Read the model definition and answer for the solid it produces. Units are mm, in the model's axes. A direction names the side the tool comes from. Give positions to 0.01 mm unless a question says otherwise; leave off trailing zeros. Order: outer loops, then holes, each group sorted by start corner. A loop starts at its lowest first (then second) coordinate and runs counter-clockwise, first axis right, second up. Notation, with made-up numbers: (2, -34) -> (47, -34) arc R15 ccw to (47, -26) -> close; hole circle Ø9 at (69.5, 20). An arc over 180 degrees is marked (long way). Answer as CSV lines item,"result". Start each with the question number.
1) Straight lines are drawn through the part: L1, parallel to Y at x = -25, z = 1.9; L2, parallel to X at y = -17, z = 1.35; L3, parallel to X at y = -18, z = 2.35. For each, find the intervals that lie inside material, in ascending order. Write a range as from..to.
2) Find section C-C (y = -26). Determine the outline of the cut face in (x, z).
3) Find section B-B (z = 2.45). State how many separate pieces and enclosed holes the cut face has, and give its area (3 significant figures).
4) Find section A-A (y = 23). Determine the outline of the cut face in (x, z).
5) Find section D-D (x = 0). Determine the outline of the cut face in (y, z), and give its area (3 significant figures).
6) For faces 1 (the face through (27.1, -26, 1)), 2 (the face through (0, -30, 1)), determine the directions among +Z, -Z, +X, -X, +Y, -Y from which every point of the face is accessible in a straight line to the end or side of a thin tool.
7) The mould has two halves that part along X. Classify faces 3 (the face through (24.65, 11.56, 1.48)), 4 (the face through (0, 30, 1)), 5 (the face through (26, -24.9, 1)), 6 (the face through (30, 0, 1)): +X half, -X half, draft (parallel to the pull), parting line (faces both ways), or undercut.
```python
from build123d import *

# Parameters (mm, degrees)
F0_W     = 60
F0_H     = 60
F1_DEPTH = 3
F2_R     = 1.6
F3_DEPTH = 3.001
F4_W     = 2.2
F4_H     = 2.2
F5_DEPTH = 3.001


with BuildPart() as f1:
    # F0 (on Top) → F1 (new body)
    with BuildSketch(Plane.XY):
        Rectangle(F0_W, F0_H)
    extrude(amount=F1_DEPTH)

    # F2 (on face) → F3 (cut, through all)
    with BuildSketch(Plane(origin=(0, 0, 0), x_dir=(1, 0, 0), z_dir=(0, 0, -1))):
        with Locations((-25, -10)):
            Circle(F2_R)
        with Locations((-25, 17)):
            Circle(F2_R)
        with Locations((25, 17)):
            Circle(F2_R)
        with Locations((25, -10)):
            Circle(F2_R)
        with Locations((0, -23)):
            Circle(F2_R)
    extrude(amount=-F3_DEPTH, mode=Mode.SUBTRACT)

    # F4 (on face) → F5 (cut, through all)
    with BuildSketch(Plane(origin=(0, 0, 0), x_dir=(1, 0, 0), z_dir=(0, 0, -1))):
        with Locations((26, 26)):
            Rectangle(F4_W, F4_H)
        with Locations((26, -26)):
            Rectangle(F4_W, F4_H)
        with Locations((-26, 26)):
            Rectangle(F4_W, F4_H)
        with Locations((-26, -26)):
            Rectangle(F4_W, F4_H)
    extrude(amount=-F5_DEPTH, mode=Mode.SUBTRACT)


solid = f1.part
```
Findings below:
1,L1,"-30..-27.1, -24.9..-18.6, -15.4..8.4, 11.6..24.9, 27.1..30"
1,L2,"-30..-26.6, -23.4..23.4, 26.6..30"
1,L3,"-30..-26.25, -23.75..23.75, 26.25..30"
2,outline,"(-30, 0) -> (-27.1, 0) -> (-27.1, 3) -> (-30, 3) -> close; (-24.9, 0) -> (24.9, 0) -> (24.9, 3) -> (-24.9, 3) -> close; (27.1, 0) -> (30, 0) -> (30, 3) -> (27.1, 3) -> close"
3,separate pieces,"1"
3,enclosed holes,"9"
3,area,"3,540 mm²"
4,outline,"(-30, 0) -> (-1.6, 0) -> (-1.6, 3) -> (-30, 3) -> close; (1.6, 0) -> (30, 0) -> (30, 3) -> (1.6, 3) -> close"
5,outline,"(-30, 0) -> (21.4, 0) -> (21.4, 3) -> (-30, 3) -> close; (24.6, 0) -> (30, 0) -> (30, 3) -> (24.6, 3) -> close"
5,area,"170 mm²"
6,face 1,"+Z, -Z"
6,face 2,"+Z, -Z, +X, -X, -Y"
7,face 3,"undercut"
7,face 4,"draft"
7,face 5,"undercut"
7,face 6,"+X half"
